Read the model definition and answer for the solid it produces. Units are mm, in the model's axes. A direction names the side the tool comes from. Give positions to 0.01 mm unless a question says otherwise; leave off trailing zeros. Order: outer loops, then holes, each group sorted by start corner. A loop starts at its lowest first (then second) coordinate and runs counter-clockwise, first axis right, second up. Notation, with made-up numbers: (29.25, 34.5) - (57.25, 34.5) arc R15 cw to (57.25, 55.5) - close; hole circle Ø4 at (52, -8). An arc over 180 degrees is marked (long way). Write item = value, one per line.
```python
from build123d import *

# Parameters (mm, degrees)
SKETCH1_R           = 1
BOSS_EXTRUDE1_DEPTH = 2
SKETCH2_W           = 26.96
SKETCH2_H           = 9.2
BOSS_EXTRUDE2_DEPTH = 6


with BuildPart() as part:
    # Sketch1 → Boss-Extrude1 (new body)
    with BuildSketch(Plane.XY):
        with BuildLine():
            Line((-15.48, -4.6), (15.48, -4.6))
            ThreePointArc((15.48, -4.6), (16.894213562, -4.014213562), (17.48, -2.6))
            Line((17.48, -2.6), (17.48, 2.6))
            ThreePointArc((17.48, 2.6), (16.894213562, 4.014213562), (15.48, 4.6))
            Line((15.48, 4.6), (-15.48, 4.6))
            ThreePointArc((-15.48, 4.6), (-16.894213562, 4.014213562), (-17.48, 2.6))
            Line((-17.48, 2.6), (-17.48, -2.6))
            ThreePointArc((-17.48, -2.6), (-16.894213562, -4.014213562), (-15.48, -4.6))
        make_face()
        with Locations((-15.48, 0)):
            Circle(SKETCH1_R, mode=Mode.SUBTRACT)
        with Locations((15.48, 0)):
            Circle(SKETCH1_R, mode=Mode.SUBTRACT)
    extrude(amount=BOSS_EXTRUDE1_DEPTH)

    # Sketch2 → Boss-Extrude2 (add)
    with BuildSketch(Plane.XY):
        Rectangle(SKETCH2_W, SKETCH2_H)
        with BuildLine():
            Line((-12.98, 4.1), (-12.98, -4.1))
            Line((-12.98, -4.1), (9.98, -4.1))
            ThreePointArc((9.98, -4.1), (12.101320344, -3.221320344), (12.98, -1.1))
            Line((12.98, -1.1), (12.98, 1.1))
            ThreePointArc((12.98, 1.1), (12.101320344, 3.221320344), (9.98, 4.1))
            Line((9.98, 4.1), (-12.98, 4.1))
        make_face(mode=Mode.SUBTRACT)
    extrude(amount=BOSS_EXTRUDE2_DEPTH)


solid = part.part
```
1. Flat-ended cylindrical pins translate along their axes: pin 1 (2 mm diameter, centred on x = 16.5, y = 2, fed in from +Z); pin 2 (1.6 mm diameter, centred on x = -15.48, y = 0, fed in from -Z); pin 3 (2 mm diameter, centred on y = -2, z = 4.5, fed in from -X); pin 4 (2 mm diameter, centred on y = 1.5, z = 4.5, fed in from +X). Find the tip coordinate at first contact, or state that the pin passes through.
Recorded:
pin_1 = 2
pin_2 = through
pin_3 = -13.48
pin_4 = 13.48
2. Section C-C (x = -9.5) is taken. Determine the outline of the cut face in (y, z), and give its area (3 significant figures).
Recorded:
outline = (-4.6, 0) - (4.6, 0) - (4.6, 6) - (4.1, 6) - (4.1, 2) - (-4.1, 2) - (-4.1, 6) - (-4.6, 6) - close
area = 22.4 mm^2
3. Section A-A (z = 0.65) is taken. Determine the outline of the cut face in (x, y).
Recorded:
outline = (-17.48, -2.6) arc R2 ccw to (-15.48, -4.6) - (15.48, -4.6) arc R2 ccw to (17.48, -2.6) - (17.48, 2.6) arc R2 ccw to (15.48, 4.6) - (-15.48, 4.6) arc R2 ccw to (-17.48, 2.6) - close; hole circle Ø2 at (-15.48, 0); hole circle Ø2 at (15.48, 0)
4. Straight lines are drawn through the part: L1, parallel to Y at x = -9.5, z = 5.6; L2, parallel to Y at x = -15.48, z = 0.75; L3, parallel to X at y = -1, z = 4.2. For each, find the intervals that lie inside material, in ascending order. Write a range as [from, to].
Recorded:
L1 = [-4.6, -4.1], [4.1, 4.6]
L2 = [-4.6, -1], [1, 4.6]
L3 = [-13.48, -12.98], [12.98, 13.48]
5. Section D-D (z = 4.8) is taken. Determine the outline of the cut face in (x, y), and give its area (3 significant figures).
Recorded:
outline = (-13.48, -4.6) - (13.48, -4.6) - (13.48, 4.6) - (-13.48, 4.6) - close; hole (-12.98, -4.1) - (9.98, -4.1) arc R3 ccw to (12.98, -1.1) - (12.98, 1.1) arc R3 ccw to (9.98, 4.1) - (-12.98, 4.1) - close
area = 39.0 mm^2
6. Determine the mould class of faces 6 (the face through (16.434, 0.3, 0.986)), 7 (the face through (-16.88, 4.03, 0.99)), 8 (the face through (0, -4.6, 3)), 9 (the face through (0, 0, 2)) for opening direction Y: +Y half, -Y half, draft (parallel to the pull), parting line (faces both ways), or undercut.
Recorded:
face_6 = undercut
face_7 = +Y half
face_8 = -Y half
face_9 = undercut
7. Section B-B (y = 0) is taken. Determine the outline of the cut face in (x, z), and give its area (3 significant figures).
Recorded:
outline = (-17.48, 0) - (-16.48, 0) - (-16.48, 2) - (-17.48, 2) - close; (-14.48, 0) - (14.48, 0) - (14.48, 2) - (13.48, 2) - (13.48, 6) - (12.98, 6) - (12.98, 2) - (-12.98, 2) - (-12.98, 6) - (-13.48, 6) - (-13.48, 2) - (-14.48, 2) - close; (16.48, 0) - (17.48, 0) - (17.48, 2) - (16.48, 2) - close
area = 65.9 mm^2
8. For faces 1 (the face through (0, 0, 0)), 2 (the face through (-13.48, 0, 4)), 3 (the face through (12.08, -3.24, 3.97)), 4 (the face through (0, 4.6, 3)), 5 (the face through (15, 1.1, 2)), determine the directions among +Z, -Z, +X, -X, +Y, -Y from which every point of the face is accessible in a straight line to the end or side of a thin tool.
Recorded:
face_1 = -Z, +X, -X, +Y, -Y
face_2 = +Z, -X, +Y, -Y
face_3 = +Z
face_4 = +Z, -Z, +X, -X, +Y
face_5 = +Z, +X, +Y, -Y
